Build history of the part. All positions in model axes, mm. Give positions to 0.01 mm unless a question says otherwise; leave off trailing zeros. Loops run counter-clockwise (first coordinate to the right, second up) from the corner with the lowest first, then second, coordinate; pieces in that order, holes last. Notation, with made-up numbers: M -24,38.25 L -8,38.25 A16 cw -8,65.25 Z; hole C 69.25,54 d8. An arc over 180 degrees is marked long. Put each result on its own line as item: value.
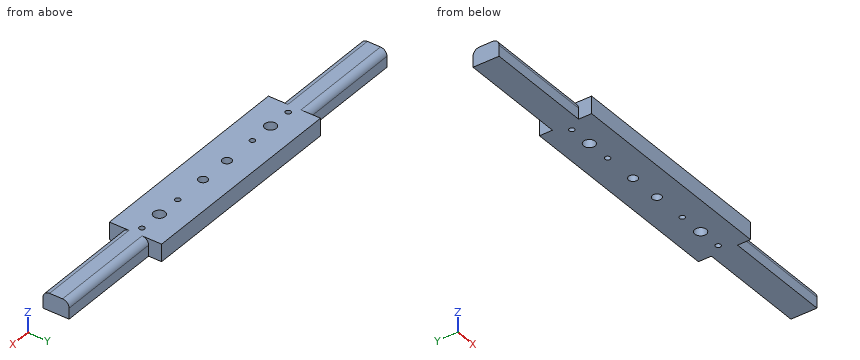
Autodesk Inventor part; units mm, degrees
ref_plane "YZ Plane" through (0, 0, 0) normal (1, 0, 0) x (0, 1, 0)
ref_plane "XZ Plane" through (0, 0, 0) normal (0, 1, 0) x (-1, 0, 0)
ref_plane "XY Plane" through (0, 0, 0) normal (0, 0, 1) x (1, 0, 0)
sketch "Sketch1" plane through (0, 0, 0) normal (0, 0, 1) x (1, 0, 0)
  line L0 (0, 20.1746) -> (0, -21.4461) construction
  line L1 (-20.2028, 0) -> (20.1685, 0) construction
  line L2 (-100, 12) -> (100, 12)
  line L3 (100, 12) -> (100, -12)
  line L4 (100, -12) -> (-100, -12)
  line L5 (-100, -12) -> (-100, 12)
  point P0 (0, 0)
  dimension "d0" = 24
  dimension "d1" = 12
  dimension "d2" = 200
  dimension "d3" = 100
extrude "Extrusion1" add sketch "Sketch1" along normal blind 8
fillet "Fillet1" [suppressed]
chamfer "Chamfer1" [suppressed]
sketch "Skizze2" plane through (0, 0, 8) normal (0, 0, 1) x (1, 0, 0)
  line L0 (-7.5, 0) -> (7.5, 0)
  point P0 (0, 0)
  point P1 (0, 0)
  dimension "d12" = 15
sketch "Skizze3" plane through (0, 0, 8) normal (0, 0, 1) x (1, 0, 0)
  line L0 (-35, 0) -> (35, 0) construction
  point P0 (0, 0)
  point P1 (0, 0)
  dimension "d13" = 70
hole "Bohrung1" at (-35, 0, 8) at (35, 0, 8) direction (0, 0, -1) diameter 5.3 end through all
hole "Bohrung2" at (-7.5, 0, 8) at (7.5, 0, 8) direction (0, 0, -1) diameter 4.134 end through all
sketch "Skizze4" plane through (0, 0, 8) normal (0, 0, 1) x (1, 0, 0)
  circle A0 centre (-46, 0) radius 1.6
  circle A1 centre (-23.5, 0) radius 1.6
  circle A2 centre (46, 0) radius 1.6
  circle A3 centre (23.5, 0) radius 1.6
  point P0 (0, 0)
hole "Bohrung3" at (23.5, 0, 8) at (46, 0, 8) at (-23.5, 0, 8) at (-46, 0, 8) direction (0, 0, -1) diameter 2.459 end through all
sketch "Skizze5" plane through (0, 0, 8) normal (0, 0, 1) x (1, 0, 0)
  line L0 (-100, 6) -> (-50, 6)
  line L1 (-50, 6) -> (-50, -6)
  line L2 (-50, -6) -> (-100, -6)
  line L3 (-100, -6) -> (-100, 6)
  line L4 (-100, 12) -> (-100, -12)
  line L5 (-50, -6) -> (-50, -12)
  line L6 (-50, 6) -> (-50, 12)
  line L7 (100, 12) -> (-100, 12)
  line L8 (-50, 12) -> (-100, 12)
  line L9 (-100, -12) -> (100, -12)
  line L10 (-50, -12) -> (-100, -12)
  line L11 (0, 12) -> (0, -12)
  line L12 (100, 6) -> (50, 6)
  line L13 (50, 6) -> (50, -6)
  line L14 (50, -6) -> (100, -6)
  line L15 (100, -6) -> (100, 6)
  line L16 (100, 12) -> (100, -12)
  line L17 (50, -6) -> (50, -12)
  line L18 (50, 6) -> (50, 12)
  line L19 (50, 12) -> (100, 12)
  line L20 (50, -12) -> (100, -12)
  point P0 (0, 0)
  point P1 (-100, 0)
  point P2 (-100, 6)
  point P3 (100, 0)
  point P4 (50, -12)
  point P5 (50, 12)
  dimension "d35" = 50
  dimension "d36" = 12
extrude "Extrusion2" cut sketch "Skizze5" against normal through all contours L4 L7 L6 L0 | L2 L5 L9 L4 | L7 L16 L12 L18 | L17 L14 L16 L9
fillet "Rundung2" radius 3 4 edges at (-75, -6, 8) (-75, 6, 8) (75, 6, 8) (75, -6, 8)
equation "\"d0\" = height"
equation "\"d1\" = 0.5 * height"
equation "\"d2\" = width"
equation "\"d3\" = 0.5 * width"
equation "\"d4\" = thickness"
equation "\"fillet\" = 0"
equation "\"chamfer\" = 0"
equation "\"thickness\" = 8"
equation "\"width\" = 200"
equation "\"height\" = 24"
properties part number "Platte Scharfe Ecken (mm) 150 x 30 x 8" material "Stahl, weich, Feste-Einspannung"
Q1. Slice it at B-B (z = 3). State how many separate pieces and enclosed holes the cut face has, and give its area (3 significant figures).
Here are the results:
separate pieces: 1
enclosed holes: 8
area: 3,510 mm²
Q2. Slice it at C-C (y = -8.75). List the corners of the cut face in (x, z).
Here are the results:
outline: M -50,0 L 50,0 L 50,8 L -50,8 Z
Q3. Drop flat-ended pins along their axis: pin 1 Ø2 at (x, y) = (46, 0) entering from -Z; pin 2 Ø7 at (x, y) = (-35, 0) entering from -Z; pin 3 Ø2.5 at (x, z) = (64, 1.5) entering from -Y; pin 4 Ø4 at (y, z) = (-8.5, 5.5) entering from +X. Give the stop position or say it passes through.
Here are the results:
pin 1: through
pin 2: z = 0
pin 3: y = -6
pin 4: x = 50
Q4. Slice it at A-A (x = -35). List the corners of the cut face in (y, z), and give its area (3 significant figures).
Here are the results:
outline: M -12,0 L -2.65,0 L -2.65,8 L -12,8 Z; M 2.65,0 L 12,0 L 12,8 L 2.65,8 Z
area: 150 mm²
Q5. Slice it at D-D (x = 64.5). List the corners of the cut face in (y, z), and give its area (3 significant figures).
Here are the results:
outline: M -6,0 L 6,0 L 6,5 A3 ccw 3,8 L -3,8 A3 ccw -6,5 Z
area: 92.1 mm²
Q6. Probe line 1 (Y direction, x = -46, z = 5.5); line 2 (Y direction, x = -7.5, z = 3.25); line 3 (X direction, y = 2.25, z = 2.75). List the from-to ranges inside material, lowest first. Write a range as from..to.
Here are the results:
line 1: -12..-1.23, 1.23..12
line 2: -12..-2.07, 2.07..12
line 3: -100..-36.4, -33.6..33.6, 36.4..100
